```python
from build123d import *

# Parameters (mm, degrees)
SKETCH1_W           = 20
SKETCH1_H           = 20
BOSS_EXTRUDE1_DEPTH = 15
SKETCH5_R           = 4.2540047
CUT_EXTRUDE1_DEPTH  = 5


with BuildPart() as part:
    # Sketch1 → Boss-Extrude1 (new body)
    with BuildSketch(Plane(origin=(0, 0, 0), x_dir=(1, 0, 0), z_dir=(0, 1, 0))):
        with Locations((10, 10)):
            Rectangle(SKETCH1_W, SKETCH1_H)
    extrude(amount=BOSS_EXTRUDE1_DEPTH)

    # Sketch4 → Cut-Revolve7 (revolve, cut)
    with BuildSketch(Plane.XY.offset(-10)):
        with BuildLine():
            Line((10, 22.5), (10, 7.5))
            ThreePointArc((10, 7.5), (17.5, 15), (10, 22.5))
        make_face()
    revolve(axis=Axis((10, 22.5, -10), (0, -1, 0)), mode=Mode.SUBTRACT)

    # Sketch5 → Cut-Extrude1 (cut)
    with BuildSketch(Plane.XZ):
        with Locations(Location((10, -10, 0), (0, 0, 270))):
            Circle(SKETCH5_R)
    extrude(amount=-CUT_EXTRUDE1_DEPTH, mode=Mode.SUBTRACT)


solid = part.part
```
Could you check a few things on this model? Use its own coordinates, in mm. Round coordinates to 2 decimals unless told otherwise and drop trailing zeros. Write each loop counter-clockwise with the first axis right and the second up, starting at its lowest first coordinate (ties: lowest second). Pieces come first, ordered by that corner, then holes.
(1) Thinking about a two-plate mould opening in Z: for faces 1 (the face through (10, 5, -10)), 2 (the face through (10, 7, -20)), 3 (the face through (8.37, 2.46, -13.93)), 4 (the face through (10, 7, 0)), which applies, +Z half, -Z half, draft (parallel to the pull), parting line (faces both ways), or undercut?
Findings below:
face 1: undercut
face 2: -Z half
face 3: undercut
face 4: +Z half
(2) Suppose I cut it at B-B on z = -10. Write out the boundary of the cut face in (x, y), and give its area (3 significant figures).
Findings below:
outline: (0, 0) - (5.75, 0) - (5.75, 5) - (14.25, 5) - (14.25, 0) - (20, 0) - (20, 15) - (17.5, 15) arc R7.5 cw to (2.5, 15) - (0, 15) - close
area: 169 mm2
(3) Suppose I cut it at C-C on x = 10. Write out the boundary of the cut face in (y, z), and give its area (3 significant figures).
Findings below:
outline: (0, -20) - (15, -20) - (15, -17.5) arc R7.5 cw to (15, -2.5) - (15, 0) - (0, 0) - (0, -5.75) - (5, -5.75) - (5, -14.25) - (0, -14.25) - close
area: 169 mm2
(4) Suppose I cut it at D-D on y = 13.5. Write out the boundary of the cut face in (x, z), and give its area (3 significant figures).
Findings below:
outline: (0, -20) - (20, -20) - (20, 0) - (0, 0) - close; hole circle Ø14.7 at (10, -10)
area: 230 mm2
(5) If I drill on probe 1 along X at (y, z) = (1.8, -10); probe 2 along Z at (x, y) = (4.75, 11.25); probe 3 along X at (y, z) = (14.25, -9), over which ranges is the centre line in solid material (lowest first)?
Findings below:
probe 1: x = 0 to 5.75, 14.25 to 20
probe 2: z = -20 to -13.82, -6.18 to 0
probe 3: x = 0 to 2.6, 17.4 to 20
(6) Suppose I cut it at A-A on y = 3.25. Write out the boundary of the cut face in (x, z).
Findings below:
outline: (0, -20) - (20, -20) - (20, 0) - (0, 0) - close; hole circle Ø8.51 at (10, -10)
(7) For pin 1 (2.5 mm diameter, centred on x = 11.5, z = -9, fed in from -Y); pin 2 (3 mm diameter, centred on x = 15.5, y = 2.5, fed in from +Z), each with a flat end and sliding along its axis, tell me the tip position at first contact or that it passes through.
Findings below:
pin 1: stops at y = 5
pin 2: stops at z = 0
